Could you check a few things on this model? Use its own coordinates, in mm. A direction names the side the tool comes from. Give positions to 0.01 mm unless a question says otherwise; leave off trailing zeros. Write each loop counter-clockwise with the first axis right and the second up, starting at its lowest first coordinate (ties: lowest second). Pieces come first, ordered by that corner, then holes. Notation, with made-up numbers: M 40,29.5 L 98,29.5 A23 cw 98,63.5 Z; hole C 5.5,-12.75 d11. An arc over 180 degrees is marked long. Use one line per item in the form item = value.
from build123d import *

# Parameters (mm, degrees)
BASE_FLANGE1_DEPTH = 7.5


# Sheet-metal steps are written as plain solids
with BuildPart() as part:
    # Sketch1 → Base-Flange1 (new, symmetric)
    with BuildSketch(Plane(origin=(0, 0, 0), x_dir=(0, 0, -1), z_dir=(1, 0, 0))):
        with BuildLine():
            Line((31.413560175, -7.925529264), (18.150160175, -7.925529264))
            ThreePointArc((18.150160175, -7.925529264), (16.922198539, -7.416890901), (16.413560175, -6.188929264))
            Line((16.413560175, -6.188929264), (16.413560175, 4.574470736))
            ThreePointArc((16.413560175, 4.574470736), (2.913560175, 18.074470736), (-10.586439825, 4.574470736))
            Line((-10.586439825, 4.574470736), (-10.586439825, -6.188929264))
            ThreePointArc((-10.586439825, -6.188929264), (-11.095078189, -7.416890901), (-12.323039825, -7.925529264))
            Line((-12.323039825, -7.925529264), (-25.586439825, -7.925529264))
            Line((-25.586439825, -7.925529264), (-25.586439825, -6.925529264))
            Line((-25.586439825, -6.925529264), (-12.323039825, -6.925529264))
            ThreePointArc((-12.323039825, -6.925529264), (-11.80218497, -6.709784119), (-11.586439825, -6.188929264))
            Line((-11.586439825, -6.188929264), (-11.586439825, 4.574470736))
            ThreePointArc((-11.586439825, 4.574470736), (2.913560175, 19.074470736), (17.413560175, 4.574470736))
            Line((17.413560175, 4.574470736), (17.413560175, -6.188929264))
            ThreePointArc((17.413560175, -6.188929264), (17.62930532, -6.709784119), (18.150160175, -6.925529264))
            Line((18.150160175, -6.925529264), (31.413560175, -6.925529264))
            Line((31.413560175, -6.925529264), (31.413560175, -7.925529264))
        make_face()
    extrude(amount=BASE_FLANGE1_DEPTH, both=True)


solid = part.part
1) If I drill on L1, parallel to Z at x = -6, y = -0.25; L2, parallel to Y at x = 2.25, z = 13.5; L3, parallel to Z at x = 0, y = 11.75, over which ranges is the centre line in solid material (lowest first)?
Checked values:
L1 = -17.41 to -16.41, 10.59 to 11.59
L2 = -7.93 to -6.93
L3 = -15.51 to -14.35, 8.52 to 9.69
2) Thinking about a two-plate mould opening in Z: for faces 1 (the flat face through (0, -1, 10.586)), 2 (the flat face through (-7.5, 10, 10)), 3 (the flat face through (0, -1, 11.586)), which applies, released by +Z, released by -Z, zero draft, split by the parting line, or undercut?
Checked values:
face_1 = undercut
face_2 = zero draft
face_3 = released by +Z
3) I want a section at B-B, the plane x = 3. Please give me the cut outline in (y, z), plus the area to 3 significant figures.
Checked values:
outline = M -7.93,-31.41 L -6.93,-31.41 L -6.93,-18.15 A0.74 cw -6.19,-17.41 L 4.57,-17.41 A14.5 ccw 4.57,11.59 L -6.19,11.59 A0.74 cw -6.93,12.32 L -6.93,25.59 L -7.93,25.59 L -7.93,12.32 A1.74 ccw -6.19,10.59 L 4.57,10.59 A13.5 cw 4.57,-16.41 L -6.19,-16.41 A1.74 ccw -7.93,-18.15 Z
area = 95.9 mm2
4) I want a section at A-A, the plane y = 0. Please give me the cut outline in (x, z), plus the area to 3 significant figures.
Checked values:
outline = M -7.5,-17.41 L 7.5,-17.41 L 7.5,-16.41 L -7.5,-16.41 Z; M -7.5,10.59 L 7.5,10.59 L 7.5,11.59 L -7.5,11.59 Z
area = 30.0 mm2
5) For faces 4 (the flat face through (7.5, 10, 10)), 5 (the flat face through (0, -6.926, 19)), 6 (the cylindrical face through (0.105, -7.43, -16.936)), 7 (the flat face through (0, -7.926, -25)), 8 (the flat face through (0, -1, -17.414)), which set-ups out of +Z, -Z, +X, -X, +Y, -Y let a thin tool reach every point of the face, with its end or its side?
Checked values:
face_4 = +Z, -Z, +X, +Y, -Y
face_5 = +Z, +X, -X, +Y
face_6 = +X, -X, -Y
face_7 = +Z, -Z, +X, -X, -Y
face_8 = -Z, +X, -X, +Y
6) I want a section at C-C, the plane z = 14. Please give me the cut outline in (x, y), plus the area to 3 significant figures.
Checked values:
outline = M -7.5,-7.93 L 7.5,-7.93 L 7.5,-6.93 L -7.5,-6.93 Z
area = 15.0 mm2
7) For pin 1 Ø3 at (x, z) = (6, -15.5) entering from -Y; pin 2 Ø5 at (y, z) = (6.5, 7) entering from +X; pin 3 Ø3 at (x, y) = (-3, -1.5) entering from +Z; pin 4 Ø6.5 at (x, z) = (3, -25.5) entering from +Y, each with a flat end and sliding along its axis, tell me the tip position at first contact or that it passes through.
Checked values:
pin_1 = -7.49
pin_2 = through
pin_3 = 11.59
pin_4 = -6.93
8) I want a section at D-D, the plane y = 6.75. Please give me the cut outline in (x, z), plus the area to 3 significant figures.
Checked values:
outline = M -7.5,-17.25 L 7.5,-17.25 L 7.5,-16.24 L -7.5,-16.24 Z; M -7.5,10.41 L 7.5,10.41 L 7.5,11.42 L -7.5,11.42 Z
area = 30.4 mm2
